The model under review builds one solid part; all positions refer to its coordinate system, in mm. Round coordinates to 2 decimals unless told otherwise and drop trailing zeros. Loops run counter-clockwise (first coordinate to the right, second up) from the corner with the lowest first, then second, coordinate; pieces in that order, holes last. Notation, with made-up numbers: (86.25, -20) -> (139.25, -20) arc R23 cw to (139.25, 13) -> close; hole circle Ø8 at (-38.5, 30.5). An arc over 180 degrees is marked (long way). Write each question's results on one line, items separated by ' | '. Start each with the question number.
Item 1: We need section A-A (y = 32.5). Give the boundary of the cut face in (x, z).
Item 2: For L1, parallel to Z at x = 0.85, y = 16; L2, parallel to Z at x = -0.3, y = 28.5; L3, parallel to X at y = 21, z = -1.55, list the stretches that pass through material, from the lowest coordinate up. Write a range as from..to.
Item 3: Mouldability with a two-part tool opening along X and no side actions: class faces 1 (the flat face through (-2, 0, 2)), 2 (the conical face through (1.745, 9.86, -0.55)), 3 (the conical face through (-0.25, 29.86, 1.11)), 4 (the cylindrical face through (-3, 19, 0)) as pulls with the +X half, pulls with the -X half, needs draft (parallel to the pull), parting line crosses it, or undercut.
Item 4: Clearance check with flat-ended pins moving along their axes: pin 1 Ø2 at (y, z) = (30, -2) entering from -X; pin 2 Ø1 at (x, y) = (-1.5, 6.5) entering from -Z; pin 3 Ø3 at (y, z) = (4.5, 1.5) entering from -X; pin 4 Ø1.5 at (y, z) = (32.5, 2.5) entering from -X. State where each tip first meets the part, or that it passes through.
Item 5: We need section B-B (y = 6.5). Give the boundary of the cut face in (x, z).
from build123d import *

# Parameters (mm, degrees)
SKETCH1_R           = 3
BOSS_EXTRUDE1_DEPTH = 40
SKETCH2_R           = 0.25
CUT_EXTRUDE1_DEPTH  = 41
CUT_EXTRUDE1_TAPER  = -3
SKETCH4_R           = 0.25
CUT_EXTRUDE3_DEPTH  = 20
CUT_EXTRUDE3_TAPER  = -5
CHAMFER2_SIZE       = 2
CHAMFER2_SIZE2      = 1.298815186


with BuildPart() as part:
    # Sketch1 → Boss-Extrude1 (new body)
    with BuildSketch(Plane(origin=(0, 0, 0), x_dir=(1, 0, 0), z_dir=(0, 1, 0))):
        Circle(SKETCH1_R)
    extrude(amount=BOSS_EXTRUDE1_DEPTH)

    # Sketch2 → Cut-Extrude1 (cut, through all)
    with BuildSketch(Plane(origin=(0, 40, 0), x_dir=(1, 0, 0), z_dir=(0, 1, 0))):
        Circle(SKETCH2_R)
    extrude(amount=-CUT_EXTRUDE1_DEPTH, taper=CUT_EXTRUDE1_TAPER, mode=Mode.SUBTRACT)

    # Sketch4 → Cut-Extrude3 (cut)
    with BuildSketch(Plane(origin=(0, 40, 0), x_dir=(1, 0, 0), z_dir=(0, 1, 0))):
        Circle(SKETCH4_R)
    extrude(amount=-CUT_EXTRUDE3_DEPTH, taper=CUT_EXTRUDE3_TAPER, mode=Mode.SUBTRACT)

    # Chamfer2
    chamfer2_edges = [part.edges().sort_by_distance(p)[0] for p in [
        (-3, 40, 0),
    ]]
    chamfer2_side = [part.faces().sort_by_distance(p)[0] for p in [
        (-3, 20, 0),
    ]]
    chamfer(chamfer2_edges, length=CHAMFER2_SIZE, length2=CHAMFER2_SIZE2, reference=chamfer2_side[0])


solid = part.part
Here are the results:
1) outline: circle Ø6 at (0, 0); hole circle Ø1.81 at (0, 0)
2) L1: z = -2.88..-1.25, 1.25..2.88 | L2: z = -2.98..-1.22, 1.22..2.98 | L3: x = -2.57..-1.12, 1.12..2.57
3) face 1: needs draft | face 2: undercut | face 3: undercut | face 4: parting line crosses it
4) pin 1: stops at x = -2.83 | pin 2: stops at z = -2.83 | pin 3: stops at x = -3 | pin 4: stops at x = -2.44
5) outline: circle Ø6 at (0, 0); hole circle Ø4.01 at (0, 0)
